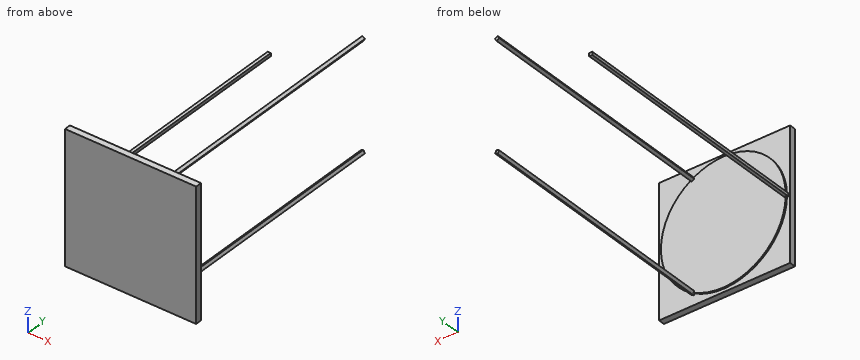
Autodesk Inventor part; units mm, degrees
ref_plane "YZ Plane" through (0, 0, 0) normal (1, 0, 0) x (0, 1, 0)
ref_plane "XZ Plane" through (0, 0, 0) normal (0, 1, 0) x (-1, 0, 0)
ref_plane "XY Plane" through (0, 0, 0) normal (0, 0, 1) x (1, 0, 0)
sketch "草圖1" plane through (0, 0, 0) normal (0, 1, 0) x (-1, 0, 0)
  circle A0 centre (0, 0) radius 200
  dimension "d0" = 400
extrude "擠出1" add sketch "草圖1" along normal blind 5
sketch "草圖2" plane through (0, 5, 0) normal (0, 1, 0) x (1, 0, 0)
  line L0 (-205, 5) -> (-195, 5)
  line L1 (-195, 5) -> (-195, -5)
  line L2 (-195, -5) -> (-205, -5)
  line L3 (-205, -5) -> (-205, 5)
  circle A0 centre (0, 0) radius 200
  line L4 (-205, 5) -> (-195, -5) construction
  line L5 (-195, 5) -> (-205, -5) construction
  point P0 (-200, 0)
  dimension "d3" = 10
  dimension "d4" = 10
extrude "擠出2" add sketch "草圖2" along normal blind 800 and the other way blind 5 contours L0 A0 L2 L3 | L0 L1 L2 A0 picked at (-196.6644, -0.5556)
pattern_circular "環形陣列1" count 3 over 360 about axis through (0, 0, 0) along (0, 1, 0) of "擠出2"
sketch "草圖3" plane through (0, 0, 0) normal (0, -1, 0) x (1, 0, 0)
  line L0 (-200, 200) -> (200, 200)
  line L1 (200, 200) -> (200, -200)
  line L2 (200, -200) -> (-200, -200)
  line L3 (-200, -200) -> (-200, 200)
  line L4 (-200, 200) -> (200, -200) construction
  line L5 (200, 200) -> (-200, -200) construction
  point P0 (0, 0)
  dimension "d12" = 400
  dimension "d13" = 400
extrude "擠出3" add sketch "草圖3" along normal blind 20
sketch "草圖4" plane through (0, -20, 0) normal (0, -1, 0) x (1, 0, 0)
  line L0 (-210, 210) -> (210, 210)
  line L1 (210, 210) -> (210, -210)
  line L2 (210, -210) -> (-210, -210)
  line L3 (-210, -210) -> (-210, 210)
  line L4 (-210, 210) -> (210, -210) construction
  line L5 (210, 210) -> (-210, -210) construction
  point P0 (0, 0)
  dimension "d16" = 420
  dimension "d17" = 420
extrude "擠出4" add sketch "草圖4" against normal up to surface (20 mm away)
properties part number "底座"
Geometry: final body of the model. Coordinates: model frame, mm. Round coordinates to 2 decimals unless told otherwise and drop trailing zeros. Order: outer loops, then holes, each group sorted by start corner. A loop starts at its lowest first (then second) coordinate and runs counter-clockwise, first axis right, second up. Notation, with made-up numbers: (33, 33) -> (89, 33) arc R7 ccw to (89, 39) -> close; hole circle Ø10 at (45, 51.25). An arc over 180 degrees is marked (long way). Use one line per item in the form item = value. Start each with the question number.
1. Cut plane A-A (y = 736). Return the cut outline in (x, z).
2. Pin query (flat end, axial travel): pin 1 Ø3 at (x, z) = (-121, 160) entering from +Y; pin 2 Ø8 at (x, y) = (-198, 269) entering from -Z; pin 3 Ø8 at (x, y) = (-202.5, 487.5) entering from +Z. Return the tip coordinate at first contact, or that it passes through.
3. Line query: probe 1 along Y at (x, z) = (114, 36.5); probe 2 along Z at (x, y) = (103, 668); probe 3 along Y at (x, z) = (-104, -189). Output: solid intervals per line, ascending.
4. Cut plane B-B (x = 65). Return the cut outline in (y, z), then the cut area to 3 significant figures.
5. Cut plane C-C (z = -105). Return the cut outline in (x, y).
Solution:
q1.outline = (-205, -5) -> (-195, -5) -> (-195, 5) -> (-205, 5) -> close; (93.17, -171.37) -> (98.17, -180.04) -> (106.83, -175.04) -> (101.83, -166.37) -> close; (93.17, 171.37) -> (101.83, 166.37) -> (106.83, 175.04) -> (98.17, 180.04) -> close
q2.pin_1 = 5
q2.pin_2 = -5
q2.pin_3 = 5
q3.probe_1 = -20 to 5
q3.probe_2 = -177.25 to -168.4, 168.4 to 177.25
q3.probe_3 = -20 to 0
q4.outline = (-20, -210) -> (0, -210) -> (0, -189.14) -> (5, -189.14) -> (5, 189.14) -> (0, 189.14) -> (0, 210) -> (-20, 210) -> close
q4.area = 10,300 mm^2
q5.outline = (-210, -20) -> (210, -20) -> (210, 0) -> (170.22, 0) -> (170.22, 5) -> (-170.22, 5) -> (-170.22, 0) -> (-210, 0) -> close
